Check sheet for the modelled part. Datum: model origin and axes. Units: mm. Face numbers are marked on the shaded views. A direction names the side the tool comes from. Round coordinates to 2 decimals unless told otherwise and drop trailing zeros. Write each loop counter-clockwise with the first axis right and the second up, starting at its lowest first coordinate (ties: lowest second). Pieces come first, ordered by that corner, then holes.
Item 1: Section check A-A, the plane x = 25. Record the cut outline in (y, z), plus the area to 3 significant figures.
Item 2: Section check D-D, the plane y = 9.75. Record the cut outline in (x, z), plus the area to 3 significant figures.
Item 3: Set-up check for the marked faces 1 and 2: record each of +Z, -Z, +X, -X, +Y, -Y from which the full face is reachable in a straight line by a thin tool's end or side.
Item 4: Release check for a two-part mould opening along Z. For the marked faces 3, 4 and 5 record: pulls with the +Z half, pulls with the -Z half, needs draft (parallel to the pull), parting line crosses it, or undercut.
Item 5: Section check C-C, the plane y = 3.25. Record the cut outline in (x, z).
Item 6: Depth check by flat-ended pin: pin 1 (12 mm diameter, centred on y = 15, z = -37.5, fed in from +X); pin 2 (10 mm diameter, centred on x = 36, z = -30, fed in from +Y). Enter the tip coordinate at first touch or a pass-through.
Item 7: Section check B-B, the plane z = -25. Record the cut outline in (x, y).
Item 8: Material ranges on line 1 along X through (y, z) = (4.75, -25); line 2 along Z through (x, y) = (25, 4.5); line 3 along Y through (x, z) = (23, -12), recorded low to high.
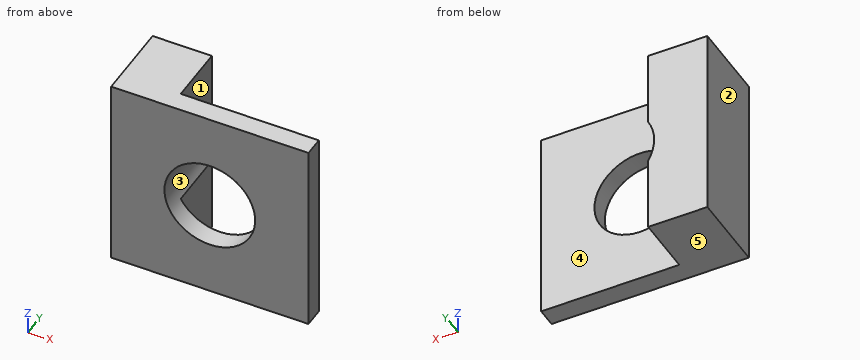
from build123d import *

# Parameters (mm, degrees)
SKETCH1_W           = 50
SKETCH1_H           = 50
BOSS_EXTRUDE1_DEPTH = 20
SKETCH2_R           = 11.5
CUT_EXTRUDE1_DEPTH  = 74.484692283
SKETCH3_W           = 38.473106937
SKETCH3_H           = 58.925618974
CUT_EXTRUDE2_DEPTH  = 15


with BuildPart() as part:
    # Sketch1 → Boss-Extrude1 (new body)
    with BuildSketch(Plane(origin=(0, 0, 0), x_dir=(1, 0, 0), z_dir=(0, 1, 0))):
        with Locations((25, 25)):
            Rectangle(SKETCH1_W, SKETCH1_H)
    extrude(amount=BOSS_EXTRUDE1_DEPTH)

    # Sketch2 → Cut-Extrude1 (cut, through all)
    with BuildSketch(Plane.XZ):
        with Locations(Location((25, -25, 0), (0, 0, 270))):
            Circle(SKETCH2_R)
    extrude(amount=-CUT_EXTRUDE1_DEPTH, mode=Mode.SUBTRACT)

    # Sketch3 → Cut-Extrude2 (cut)
    with BuildSketch(Plane(origin=(0, 20, 0), x_dir=(1, 0, 0), z_dir=(0, 1, 0))):
        with Locations((34.236553469, 26.583369284)):
            Rectangle(SKETCH3_W, SKETCH3_H)
    extrude(amount=-CUT_EXTRUDE2_DEPTH, mode=Mode.SUBTRACT)


solid = part.part
Values found:
1. outline: (0, -50) - (5, -50) - (5, -36.5) - (0, -36.5) - close; (0, -13.5) - (5, -13.5) - (5, 0) - (0, 0) - close
1. area: 135 mm2
2. outline: (0, -50) - (15, -50) - (15, -30.68) arc R11.5 cw to (15, -19.32) - (15, 0) - (0, 0) - close
2. area: 738 mm2
3. face 1: +Z, -Z, +X, +Y
3. face 2: +Z, -Z, -X, +Y, -Y
4. face 3: undercut
4. face 4: needs draft
4. face 5: pulls with the -Z half
5. outline: (0, -50) - (50, -50) - (50, 0) - (0, 0) - close; hole circle Ø23 at (25, -25)
6. pin 1: stops at x = 15
6. pin 2: stops at y = 5
7. outline: (0, 0) - (13.5, 0) - (13.5, 20) - (0, 20) - close; (36.5, 0) - (50, 0) - (50, 5) - (36.5, 5) - close
8. line 1: x = 0 to 13.5, 36.5 to 50
8. line 2: z = -50 to -36.5, -13.5 to 0
8. line 3: y = 0 to 5
